Design review of the part built by this model. Coordinates are the model's own, in mm. A direction names the side the tool comes from. Coordinates: 2 decimals unless noted, no trailing zeros. Write each loop counter-clockwise with the first axis right and the second up, starting at its lowest first coordinate (ties: lowest second). Pieces come first, ordered by that corner, then holes. Notation, with made-up numbers: (-8, 13) - (33, 13) arc R15 ccw to (33, 25) - close; hole circle Ø10 at (-34.75, -28). An arc over 180 degrees is marked (long way). Answer as a JSON object with one key per item and string values.
```python
from build123d import *

# Parameters (mm, degrees)
CROQUIS1_R            = 9.12
CROQUIS1_R_2          = 6.5
EXTRUIR_L_MINA1_DEPTH = 20.62
CROQUIS2_W            = 2.36
CROQUIS2_H            = 20
CORTAR_EXTRUIR1_DEPTH = 3.25


with BuildPart() as part:
    # Croquis1 → Extruir-Lámina1 (new body)
    with BuildSketch(Plane.XY):
        Circle(CROQUIS1_R)
        Circle(CROQUIS1_R_2, mode=Mode.SUBTRACT)
    extrude(amount=-EXTRUIR_L_MINA1_DEPTH)

    # Croquis2 → Cortar-Extruir1 (cut)
    with BuildSketch(Plane.XY):
        Rectangle(CROQUIS2_W, CROQUIS2_H)
    extrude(amount=-CORTAR_EXTRUIR1_DEPTH, mode=Mode.SUBTRACT)


solid = part.part
```
(1) Tool access review of faces 1 (the face through (1.18, -8, -2)), 2 (the face through (-1.409, -6.345, -10.166)): name each direction out of +Z, -Z, +X, -X, +Y, -Y from which nothing blocks a thin tool from reaching the whole face with its end or side.
Solved:
{"face 1": "+Z, +Y, -Y", "face 2": "+Z, -Z"}
(2) Take a section at D-D, the plane y = -7.5. Write out the cut boundary in (x, z), and give its area (3 significant figures).
Solved:
{"outline": "(-5.19, -20.62) - (5.19, -20.62) - (5.19, 0) - (1.18, 0) - (1.18, -3.25) - (-1.18, -3.25) - (-1.18, 0) - (-5.19, 0) - close", "area": "206 mm^2"}
(3) To check wall thickness, follow line 1 (X direction, y = 0, z = -12.5); line 2 (X direction, y = -8, z = -2.75). State the ranges of each line that lie inside material, in increasing order. Write a range as from..to.
Solved:
{"line 1": "x = -9.12..-6.5, 6.5..9.12", "line 2": "x = -4.38..-1.18, 1.18..4.38"}
(4) The part is to be moulded in two halves that separate along X. For faces 3 (the face through (-7.237, -5.549, -10.166)), 4 (the face through (-7, 0, 0)), 5 (the face through (1.18, 8, -2)), say which applies: pulls with the +X half, pulls with the -X half, needs draft (parallel to the pull), parting line crosses it, or undercut.
Solved:
{"face 3": "parting line crosses it", "face 4": "needs draft", "face 5": "undercut"}
(5) Take a section at C-C, the plane z = -14.25. Write out the cut boundary in (x, y), and give its area (3 significant figures).
Solved:
{"outline": "circle Ø18.24 at (0, 0); hole circle Ø13 at (0, 0)", "area": "129 mm^2"}
(6) Take a section at A-A, the plane y = 0. Write out the cut boundary in (x, z), and give its area (3 significant figures).
Solved:
{"outline": "(-9.12, -20.62) - (-6.5, -20.62) - (-6.5, 0) - (-9.12, 0) - close; (6.5, -20.62) - (9.12, -20.62) - (9.12, 0) - (6.5, 0) - close", "area": "108 mm^2"}
(7) For pin 1 (0.8 mm diameter, centred on y = -7.5, z = -2, fed in from +X); pin 2 (3 mm diameter, centred on y = 8, z = -1, fed in from -X); pin 3 (0.8 mm diameter, centred on y = -7.5, z = -2.5, fed in from -X); pin 4 (4 mm diameter, centred on x = 3, y = 2.5, fed in from +Z), all flat-tipped, find the tip position at first contact; note any pin that passes through.
Solved:
{"pin 1": "stops at x = 5.72", "pin 2": "stops at x = -6.4", "pin 3": "stops at x = -5.72", "pin 4": "passes through"}
(8) Take a section at B-B, the plane x = 0. Write out the cut boundary in (y, z), and give its area (3 significant figures).
Solved:
{"outline": "(-9.12, -20.62) - (-6.5, -20.62) - (-6.5, -3.25) - (-9.12, -3.25) - close; (6.5, -20.62) - (9.12, -20.62) - (9.12, -3.25) - (6.5, -3.25) - close", "area": "91.0 mm^2"}
